Check sheet for the modelled part. Datum: model origin and axes. Units: mm. A direction names the side the tool comes from. Coordinates: 2 decimals unless noted, no trailing zeros. Order: outer loops, then holes, each group sorted by start corner. A loop starts at its lowest first (then second) coordinate and runs counter-clockwise, first axis right, second up.
Autodesk Inventor part; units mm, degrees
ref_plane "YZ Plane" through (0, 0, 0) normal (1, 0, 0) x (0, 1, 0)
ref_plane "XZ Plane" through (0, 0, 0) normal (0, 1, 0) x (-1, 0, 0)
ref_plane "XY Plane" through (0, 0, 0) normal (0, 0, 1) x (1, 0, 0)
sketch "Sketch1" plane through (0, 0, 0) normal (0, 1, 0) x (-1, 0, 0)
  line L0 (0, 0) -> (152.4, 0) construction
  line L1 (152.4, 0) -> (152.4, -152.4) construction
  line L2 (152.4, -152.4) -> (0, -152.4) construction
  line L3 (0, -152.4) -> (0, 0) construction
  line L4 (44.6369, -152.4) -> (0, -107.7631)
  line L5 (0, -107.7631) -> (0, -44.6369)
  line L6 (0, -44.6369) -> (44.6369, 0)
  line L7 (44.6369, 0) -> (107.7631, 0)
  line L8 (107.7631, 0) -> (152.4, -44.6369)
  line L9 (152.4, -44.6369) -> (152.4, -107.7631)
  line L10 (152.4, -107.7631) -> (107.7631, -152.4)
  line L11 (107.7631, -152.4) -> (44.6369, -152.4)
  line L12 (102.5026, -12.7) -> (139.7, -49.8974)
  line L13 (139.7, -49.8974) -> (139.7, -102.5026)
  line L14 (139.7, -102.5026) -> (102.5026, -139.7)
  line L15 (102.5026, -139.7) -> (49.8974, -139.7)
  line L16 (49.8974, -139.7) -> (12.7, -102.5026)
  line L17 (12.7, -102.5026) -> (12.7, -49.8974)
  line L18 (12.7, -49.8974) -> (49.8974, -12.7)
  line L19 (49.8974, -12.7) -> (102.5026, -12.7)
  point P0 (76.2, -76.2)
  point P1 (76.2, -76.2)
  point P2 (76.2, -76.2)
  dimension "d0" = 152.4
  dimension "d1" = 152.4
  dimension "d2" = 12.7
  dimension "d3" = 63.1262
  dimension "d4" = 52.6051
sketch "Sketch2" plane through (0, 0, 0) normal (0, 1, 0) x (-1, 0, 0)
  line L0 (0, 0) -> (152.4, 0) construction
  line L1 (152.4, 0) -> (152.4, -152.4) construction
  line L2 (152.4, -152.4) -> (0, -152.4) construction
  line L3 (0, -152.4) -> (0, 0) construction
  line L4 (44.6369, -152.4) -> (0, -107.7631)
  line L5 (0, -107.7631) -> (0, -44.6369)
  line L6 (0, -44.6369) -> (44.6369, 0)
  line L7 (44.6369, 0) -> (107.7631, 0)
  line L8 (107.7631, 0) -> (152.4, -44.6369)
  line L9 (152.4, -44.6369) -> (152.4, -107.7631)
  line L10 (152.4, -107.7631) -> (107.7631, -152.4)
  line L11 (107.7631, -152.4) -> (44.6369, -152.4)
  line L12 (102.5026, -12.7) -> (139.7, -49.8974)
  line L13 (139.7, -49.8974) -> (139.7, -102.5026)
  line L14 (139.7, -102.5026) -> (102.5026, -139.7)
  line L15 (102.5026, -139.7) -> (49.8974, -139.7)
  line L16 (49.8974, -139.7) -> (12.7, -102.5026)
  line L17 (12.7, -102.5026) -> (12.7, -49.8974)
  line L18 (12.7, -49.8974) -> (49.8974, -12.7)
  line L19 (49.8974, -12.7) -> (102.5026, -12.7)
  point P0 (76.2, -76.2)
  point P1 (76.2, -76.2)
  point P2 (76.2, -76.2)
  dimension "d5" = 152.4
  dimension "d6" = 152.4
  dimension "d7" = 12.7
  dimension "d8" = 63.1262
  dimension "d9" = 52.6051
extrude "Extrusion1" add sketch "Sketch1" along normal blind 12.7 contours L4 L5 L6 L7 L8 L9 L10 L11 | L12 L13 L14 L15 L16 L17 L18 L19
extrude "Extrusion2" add sketch "Sketch2" along normal blind 19.05 contours L12 L13 L14 L15 L16 L17 L18 L19
properties part number "SatelliteTopFace"
(1) Go/stop test with flat-tipped pins: P1, Ø1.5, axis at x = -44.5, y = 15, coming from the +Z side; P2, Ø3, axis at y = 15, z = -51, coming from the +X side; P3, Ø1, axis at y = 4.5, z = -39.5, coming from the +X side. Record where each tip stops, or that it passes through.
Filled in:
P1: stops at z = -17.35
P2: stops at x = -12.7
P3: stops at x = -4.64
(2) Tool access check on faces 1 (the flat face through (-77, 16, -139.7)), 2 (the flat face through (-31, 15.8, -31.6)), 3 (the flat face through (-139.7, 16, -76)). Record the directions out of +Z, -Z, +X, -X, +Y, -Y that give a thin tool (end or side, any length) a straight path to the whole face; none if there is none.
Filled in:
face 1: -Z, +X, -X, +Y
face 2: +Z, +X, +Y
face 3: +Z, -Z, -X, +Y
(3) Cross-section at A-A (y = 3). Enter the section's corners in (x, z).
Filled in:
outline: (-152.4, -107.76) - (-107.76, -152.4) - (-44.64, -152.4) - (0, -107.76) - (0, -44.64) - (-44.64, 0) - (-107.76, 0) - (-152.4, -44.64) - close
(4) Cross-section at B-B (x = -90). Enter the section's corners in (y, z), and give its area (3 significant figures).
Filled in:
outline: (0, -152.4) - (12.7, -152.4) - (12.7, -139.7) - (19.05, -139.7) - (19.05, -12.7) - (12.7, -12.7) - (12.7, 0) - (0, 0) - close
area: 2,740 mm2
(5) Thickness scan on probe 1 along Z at (x, y) = (-62.5, 17.75); probe 2 along Y at (x, z) = (-10, -85.5); probe 3 along X at (y, z) = (9, -117.5). Record the ranges inside material, lowest first.
Filled in:
probe 1: z = -139.7 to -12.7
probe 2: y = 0 to 12.7
probe 3: x = -142.66 to -9.74
